Geometry check sheet. Reference: the model listing, model coordinates, mm. Face numbers are marked on the shaded views. A direction names the side the tool comes from. Give positions to 0.01 mm unless a question says otherwise; leave off trailing zeros. Loops run counter-clockwise (first coordinate to the right, second up) from the corner with the lowest first, then second, coordinate; pieces in that order, holes last. Notation, with made-up numbers: (82, 32.5) - (137, 32.5) arc R27 cw to (137, 63.5) - close; hole circle Ø8 at (40.5, 52). An arc over 180 degrees is marked (long way). One line per question, with ' | ' between items. Start each with the question number.
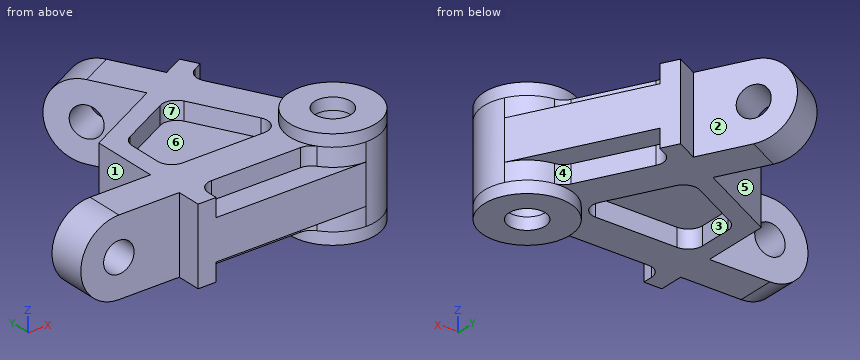
from build123d import *
from build123d.topology import SkipClean

# Parameters (mm, degrees)
SKETCH2_R            = 8
BOSS_EXTRUDE1_DEPTH  = 9.75
SKETCH3_R            = 8
BOSS_EXTRUDE2_DEPTH  = 9.75
SKETCH5_R            = 22.5
BOSS_EXTRUDE3_DEPTH  = 20
SKETCH6_R            = 9.5
CUT_EXTRUDE1_DEPTH   = 20
CUT_EXTRUDE3_DEPTH   = 9.5
FILLET1_R            = 7.5
FILLET1_OF_MIRROR1_R = 7.5
BOSS_EXTRUDE5_START  = 6.35
SKETCH9_R            = 22.5
SKETCH9_R_2          = 9.5
BOSS_EXTRUDE5_DEPTH  = 6.35


with BuildPart() as part:
    # Sketch2 → Boss-Extrude1 (new, symmetric)
    with BuildSketch(Plane(origin=(0, 0, 0), x_dir=(1, 0, 0), z_dir=(0, 1, 0))):
        with BuildLine():
            Line((0, -20), (-120, -20))
            ThreePointArc((-120, -20), (-140, 0), (-120, 20))
            Line((-120, 20), (0, 20))
            Line((0, 20), (0, -20))
        make_face()
        with Locations(Location((-120, 0, 0), (0, 0, 270))):
            Circle(SKETCH2_R, mode=Mode.SUBTRACT)
    extrude(amount=BOSS_EXTRUDE1_DEPTH, both=True)

    # Sketch3 → Boss-Extrude2 (add, symmetric)
    with BuildSketch(Plane(origin=(0, 0, 0), x_dir=(0.46174861323503175, -0.8870108331782229, 0), z_dir=(0.8870108331782228, 0.4617486132350317, 0))):
        with BuildLine():
            Line((0, -20), (-108, -20))
            ThreePointArc((-108, -20), (-128, 0), (-108, 20))
            Line((-108, 20), (0, 20))
            Line((0, 20), (0, -20))
        make_face()
        with Locations(Location((-108, 0, 0), (0, 0, 180))):
            Circle(SKETCH3_R, mode=Mode.SUBTRACT)
    extrude(amount=BOSS_EXTRUDE2_DEPTH, both=True)

    # Sketch5 → Boss-Extrude3 (add, symmetric)
    with BuildSketch(Plane.XY):
        with BuildLine():
            Line((-88.25, -22.5), (0, -22.5))
            ThreePointArc((0, -22.5), (-19.23551709, 11.672398309), (19.957743747, 10.389343798))
            Line((19.957743747, 10.389343798), (-17.18672299, 81.743200515))
            Line((-17.18672299, 81.743200515), (-88.25, 44.75))
            Line((-88.25, 44.75), (-88.25, -22.5))
        make_face()
        Circle(SKETCH5_R)
    extrude(amount=BOSS_EXTRUDE3_DEPTH, both=True)

    # Sketch6 → Cut-Extrude1 (cut, symmetric)
    with BuildSketch(Plane.XY):
        Circle(SKETCH6_R)
    extrude(amount=CUT_EXTRUDE1_DEPTH, both=True, mode=Mode.SUBTRACT)

    # Sketch7 → Cut-Extrude3 (cut)
    with BuildSketch(Plane.XY.offset(20)):
        with BuildLine():
            Line((-78.75, -22.5), (0, -22.5))
            ThreePointArc((0, -22.5), (-11.976539567, -19.047637649), (-20.277758752, -9.75))
            Line((-20.277758752, -9.75), (-78.75, -9.75))
            Line((-78.75, -9.75), (-78.75, -22.5))
        make_face()
        with BuildLine():
            Line((-12.800111165, 73.3165976), (-24.109499288, 67.429302781))
            Line((-24.109499288, 67.429302781), (-0.71487136, 22.488640665))
            ThreePointArc((-0.71487136, 22.488640665), (11.365310405, 19.41854061), (19.957743747, 10.389343798))
            Line((19.957743747, 10.389343798), (-12.800111165, 73.3165976))
        make_face()
        Polygon((-16.067502725, 9.75), (-41.406210535, 58.425204823), (-78.75, 38.985258485), (-78.75, 9.75), align=None)
    cut_extrude3 = extrude(amount=-CUT_EXTRUDE3_DEPTH, mode=Mode.SUBTRACT)

    # Fillet1
    fillet1_edges = [part.edges().sort_by_distance(p)[0] for p in [
        (-20.277758752, -9.75, 15.25),
        (-78.75, -9.75, 15.25),
        (-78.75, 38.985258485, 15.25),
        (-41.406210535, 58.425204823, 15.25),
        (-16.067502725, 9.75, 15.25),
        (-78.75, 9.75, 15.25),
        (-0.71487136, 22.488640665, 15.25),
        (-24.109499288, 67.429302781, 15.25),
    ]]
    fillet(fillet1_edges, radius=FILLET1_R)

    # Mirror1: Cut-Extrude3 across plane
    add(cut_extrude3.mirror(Plane.XY), mode=Mode.SUBTRACT)

    # Fillet1 of Mirror1
    fillet1_of_mirror1_edges = [part.edges().sort_by_distance(p)[0] for p in [
        (-20.277758752, -9.75, -15.25),
        (-78.75, -9.75, -15.25),
        (-78.75, 38.985258485, -15.25),
        (-41.406210535, 58.425204823, -15.25),
        (-16.067502725, 9.75, -15.25),
        (-78.75, 9.75, -15.25),
        (-0.71487136, 22.488640665, -15.25),
        (-24.109499288, 67.429302781, -15.25),
    ]]
    fillet(fillet1_of_mirror1_edges, radius=FILLET1_OF_MIRROR1_R)

    # Sketch9 → Boss-Extrude5 (add)
    with SkipClean():  # the faces are left unmerged after this step: merging them gives an invalid solid
        with BuildSketch(Plane.XY.offset(20).offset(BOSS_EXTRUDE5_START)):
            with Locations(Location((0, 0, 0), (0, 0, 215.099632195))):
                Circle(SKETCH9_R)
            Circle(SKETCH9_R_2, mode=Mode.SUBTRACT)
        boss_extrude5 = extrude(amount=-BOSS_EXTRUDE5_DEPTH)

    # Mirror2: Boss-Extrude5 across plane
    with SkipClean():  # the faces are left unmerged after this step: merging them gives an invalid solid
        add(boss_extrude5.mirror(Plane.XY))


solid = part.part
(1) Section check B-B, the plane z = 0. Record the boundary of the cut face in (x, y), and give its area (3 significant figures).
(2) Section check C-C, the plane y = 78.5. Record the boundary of the cut face in (x, z).
(3) Section check A-A, the plane y = 0. Record the boundary of the cut face in (x, z).
(4) Mould release check, pull along X, two halves, no side actions. Record for the marked faces 4, 5, 6 and 7: pulls with the +X half, pulls with the -X half, needs draft (parallel to the pull), parting line crosses it, or undercut.
(5) Material ranges on line 1 (Y direction, x = 0, z = -23.5); line 2 (Z direction, x = -11.5, y = 52); line 3 (X direction, y = 19.5, z = 12.5), recorded low to high.
(6) Section check D-D, the plane x = -122. Record the boundary of the cut face in (y, z), and give its area (3 significant figures).
(7) Depth check by flat-ended pin: pin 1 Ø6 at (y, z) = (7.5, 20) entering from -X; pin 2 Ø7.5 at (x, z) = (-46.5, -16) entering from -Y; pin 3 Ø17 at (x, y) = (0, 0) entering from +Z; pin 4 Ø3 at (x, z) = (-108.5, -20) entering from +Y. Enter the tip coordinate at first touch or a pass-through.
(8) Tool access check on the marked faces 1, 2 and 3. Record the directions out of +Z, -Z, +X, -X, +Y, -Y that give a thin tool (end or side, any length) a straight path to the whole face; none if there is none.
Numbers:
1) outline: (-140, -9.75) - (-128, -9.75) - (-128, 9.75) - (-140, 9.75) - close; (-112, -9.75) - (-88.25, -9.75) - (-88.25, -22.5) - (0, -22.5) arc R22.5 ccw to (19.96, 10.39) - (-17.19, 81.74) - (-28.5, 75.86) - (-37.53, 93.2) - (-54.82, 84.2) - (-45.79, 66.85) - (-88.25, 44.75) - (-88.25, 9.75) - (-112, 9.75) - close; (-67.75, 109.04) - (-62.21, 98.39) - (-44.91, 107.4) - (-50.46, 118.04) - close; hole circle Ø19 at (0, 0) | area: 9,640 mm^2
2) outline: (-51.86, -20) - (-29.87, -20) - (-29.87, 20) - (-51.86, 20) - close; (-23.42, -20) - (-15.5, -20) - (-15.5, 20) - (-23.42, 20) - close
3) outline: (-120, -20) - (-22.5, -20) - (-22.5, -26.35) - (-9.5, -26.35) - (-9.5, 26.35) - (-22.5, 26.35) - (-22.5, 20) - (-120, 20) arc R20 ccw to start; (9.5, -26.35) - (22.5, -26.35) - (22.5, 26.35) - (9.5, 26.35) - close; hole circle Ø16 at (-120, 0)
4) face 4: pulls with the +X half | face 5: pulls with the -X half | face 6: undercut | face 7: undercut
5) line 1: -22.5 to -9.5, 9.5 to 22.5 | line 2: -10.5 to 10.5 | line 3: -88.25 to -78.75, -21.27 to 11.22
6) outline: (-9.75, -19.9) - (9.75, -19.9) - (9.75, -7.75) - (-9.75, -7.75) - close; (-9.75, 7.75) - (9.75, 7.75) - (9.75, 19.9) - (-9.75, 19.9) - close | area: 474 mm^2
7) pin 1: x = -130.54 | pin 2: y = -9.75 | pin 3: through | pin 4: y = 9.75
8) face 1: +Z, -Z, -X, +Y | face 2: +Z, -Z, +Y | face 3: -Z
